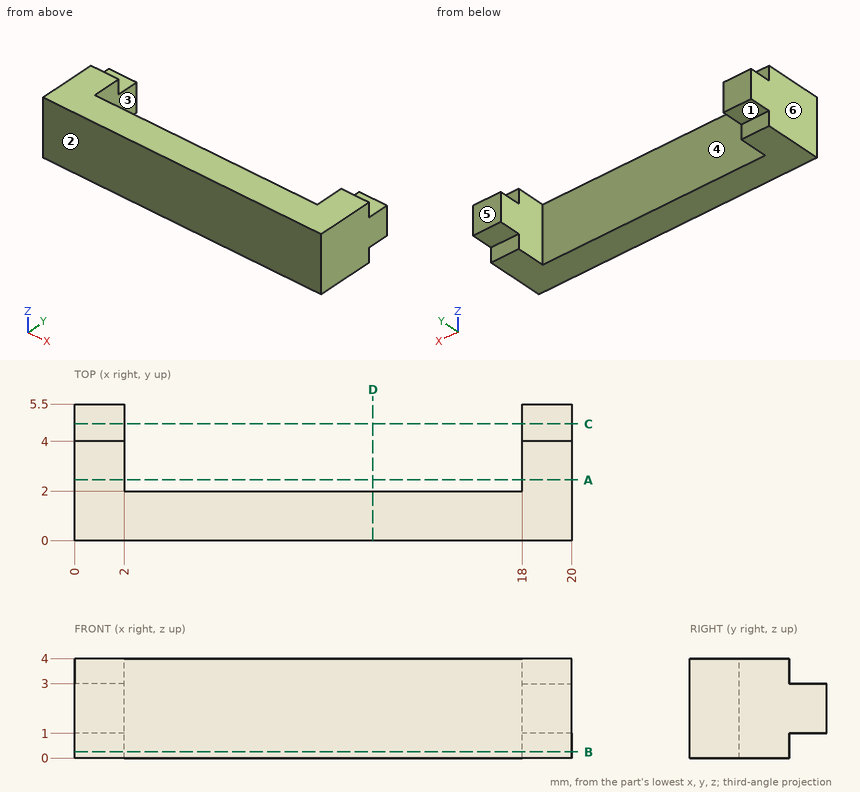
Geometry: see drawing. Coordinates: mm, zero at the bounding-box minimum. A direction names the side the tool comes from. Coordinates: 2 decimals unless noted, no trailing zeros. Loops run counter-clockwise (first coordinate to the right, second up) from the corner with the lowest first, then second, coordinate; pieces in that order, holes last. Notation, with made-up numbers: (73.5, 18) -> (114.5, 18) arc R19 cw to (114.5, 31) -> close; hole circle Ø5 at (-17.5, 54.5). An arc over 180 degrees is marked (long way). Use a Markdown table: item, result.
1) Material intervals for line 1 along X through (y, z) = (3, 3.4); line 2 along Y through (x, z) = (3.75, 3.25); line 3 along Y through (x, z) = (19.25, 0.5), sorted ascending. Write a range as from..to.
Results found:
| item | result |
|---|---|
| line 1 | x = 0..2, 18..20 |
| line 2 | y = 0..2 |
| line 3 | y = 0..4 |
2) Cut plane B-B (z = 0.25). Return the cut outline in (x, y).
Results found:
| item | result |
|---|---|
| outline | (0, 0) -> (20, 0) -> (20, 4) -> (18, 4) -> (18, 2) -> (2, 2) -> (2, 4) -> (0, 4) -> close |
3) Cut plane C-C (y = 4.7). Return the cut outline in (x, z), then the cut area to 3 significant figures.
Results found:
| item | result |
|---|---|
| outline | (0, 1) -> (2, 1) -> (2, 3) -> (0, 3) -> close; (18, 1) -> (20, 1) -> (20, 3) -> (18, 3) -> close |
| area | 8.00 mm2 |
4) Cut plane D-D (x = 12). Return the cut outline in (y, z), then the cut area to 3 significant figures.
Results found:
| item | result |
|---|---|
| outline | (0, 0) -> (2, 0) -> (2, 4) -> (0, 4) -> close |
| area | 8.00 mm2 |
5) Contact query for flat-ended pins moving along their axis: pin 1 (0.8 mm diameter, centred on x = 19, y = 4.5, fed in from +Z); pin 2 (1.6 mm diameter, centred on x = 1, y = 5, fed in from -Z); pin 3 (0.8 mm diameter, centred on x = 19.5, z = 0.5, fed in from +Y). Output: stop coordinate, or through.
Results found:
| item | result |
|---|---|
| pin 1 | stops at z = 3 |
| pin 2 | stops at z = 1 |
| pin 3 | stops at y = 4 |
6) Cut plane A-A (y = 2.45). Return the cut outline in (x, z), then the cut area to 3 significant figures.
Results found:
| item | result |
|---|---|
| outline | (0, 0) -> (2, 0) -> (2, 4) -> (0, 4) -> close; (18, 0) -> (20, 0) -> (20, 4) -> (18, 4) -> close |
| area | 16.0 mm2 |
7) Pull-direction query (X, two-part tool) for the marked faces 4, 5 and 6; classes: released by +X, released by -X, zero draft, split by the parting line, or undercut.
Results found:
| item | result |
|---|---|
| face 4 | undercut |
| face 5 | zero draft |
| face 6 | released by -X |
8) Access query for the marked faces 1, 2 and 3. Directions: +Z, -Z, +X, -X, +Y, -Y. A direction counts if a zero-diameter tool reaches every point of the face in a straight line with its end or side. Return the directions, or none.
Results found:
| item | result |
|---|---|
| face 1 | -Z, +X, -X, +Y |
| face 2 | +Z, -Z, +X, -X, -Y |
| face 3 | +Z, -Z, +Y |
